Answer from the drawing. Dimensions are ordinates in mm from the lowest x, y and z of the part. A direction names the side the tool comes from. Coordinates: 2 decimals unless noted, no trailing zeros. Write each loop counter-clockwise with the first axis right and the second up, starting at its lowest first coordinate (ties: lowest second). Pieces come first, ordered by that corner, then holes.
(1) Section D-D on y = 16 is taken. Write down the section's boundary in (x, z).
(2) Given pin 1 (3 mm diameter, centred on y = 27.5, z = 27.5, fed in from +X); pin 2 (4 mm diameter, centred on y = 32.8, z = 12.5, fed in from -X); pin 3 (4 mm diameter, centred on x = 26, y = 22.5, fed in from -Z), each flat-ended and moving along its own axis, determine where each tip first touches the part or whether it passes through.
(3) Section A-A on z = 12.5 is taken. Write down the section's boundary in (x, y).
(4) Which of the six approach directions +Z, -Z, +X, -X, +Y, -Y give full straight-line access (tool end or side, diameter ignored) to the marked faces 1 and 2?
(5) Section C-C on y = 7.8 is taken. Write down the section's boundary in (x, z), then the cut area to 3 significant figures.
(6) Find the intervals of material crossed by probe 1 along Y at (x, z) = (2.55, 12.5); probe 2 along X at (y, z) = (5.3, 50.35); probe 3 along Z at (x, y) = (2.7, 7.8), in increasing order.
(7) Section B-B on x = 25.5 is taken. Write down the section's boundary in (y, z), then the cut area to 3 significant figures.
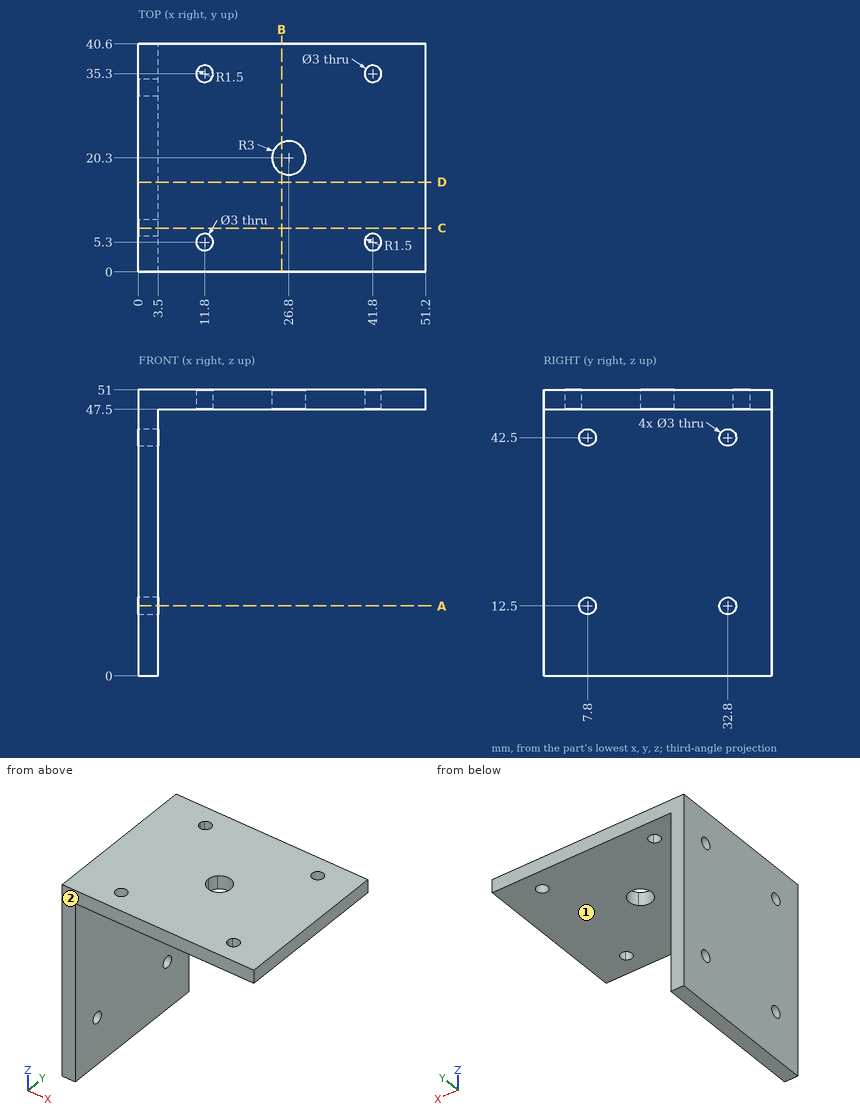
Response:
1. outline: (0, 0) - (3.5, 0) - (3.5, 47.5) - (51.2, 47.5) - (51.2, 51) - (0, 51) - close
2. pin 1: stops at x = 3.5
2. pin 2: stops at x = 0
2. pin 3: stops at z = 47.5
3. outline: (0, 0) - (3.5, 0) - (3.5, 6.3) - (0, 6.3) - close; (0, 9.3) - (3.5, 9.3) - (3.5, 31.3) - (0, 31.3) - close; (0, 34.3) - (3.5, 34.3) - (3.5, 40.6) - (0, 40.6) - close
4. face 1: -Z, +X, +Y, -Y
4. face 2: +Z, -Z, +X, -X, -Y
5. outline: (0, 0) - (3.5, 0) - (3.5, 11) - (0, 11) - close; (0, 14) - (3.5, 14) - (3.5, 41) - (0, 41) - close; (0, 44) - (3.5, 44) - (3.5, 47.5) - (51.2, 47.5) - (51.2, 51) - (0, 51) - close
5. area: 324 mm2
6. probe 1: y = 0 to 6.3, 9.3 to 31.3, 34.3 to 40.6
6. probe 2: x = 0 to 10.3, 13.3 to 40.3, 43.3 to 51.2
6. probe 3: z = 0 to 11, 14 to 41, 44 to 51
7. outline: (0, 47.5) - (17.6, 47.5) - (17.6, 51) - (0, 51) - close; (23, 47.5) - (40.6, 47.5) - (40.6, 51) - (23, 51) - close
7. area: 123 mm2
